For this review, use the dimensioned drawing (mm, ordinates from the lowest corner) and the shaded views. A direction names the side the tool comes from. Round coordinates to 2 decimals unless told otherwise and drop trailing zeros. Order: outer loops, then holes, each group sorted by start corner. A loop starts at its lowest first (then second) coordinate and runs counter-clockwise, first axis right, second up. Notation, with made-up numbers: M 12.25,83 L 70.25,83 A23 ccw 70.25,120 Z; hole C 1.25,-31 d7. An arc over 180 degrees is marked long. Use a Markdown table: item, result. Add a question column.
1. Consider section A-A on z = 4.15. State the section outline as (x, y) points (1 decimal), then the cut area to 3 significant figures.
2. Consider section B-B on z = 0.8. State the section outline as (x, y) points (1 decimal), then the cut area to 3 significant figures.
3. The part is to be moulded in two halves that separate along X. For the marked faces 3, 4 and 5, say which applies: +X half, -X half, draft (parallel to the pull), parting line (faces both ways), or undercut.
4. For the marked faces 1 and 2, list the 3-axis set-ups (+Z, -Z, +X, -X, +Y, -Y) from which the entire face can be reached by the end or side of a thin tool; tool diameter is ignored.
5. To check wall thickness, follow probe 1 along Y at (x, z) = (11, 4.3); probe 2 along Z at (x, y) = (9.75, 2) (1 decimal). State the ranges of each line that lie inside material, in increasing order.
6. Insertion check: P1, Ø1.5, axis at y = 5.5, z = 2.5, coming from the -X side; P2, Ø2, axis at x = 5.5, y = 11.5, coming from the +Z side. Each pin has a flat end and moves straight along its axis. Give the tip position at first contact, or say it passes through.
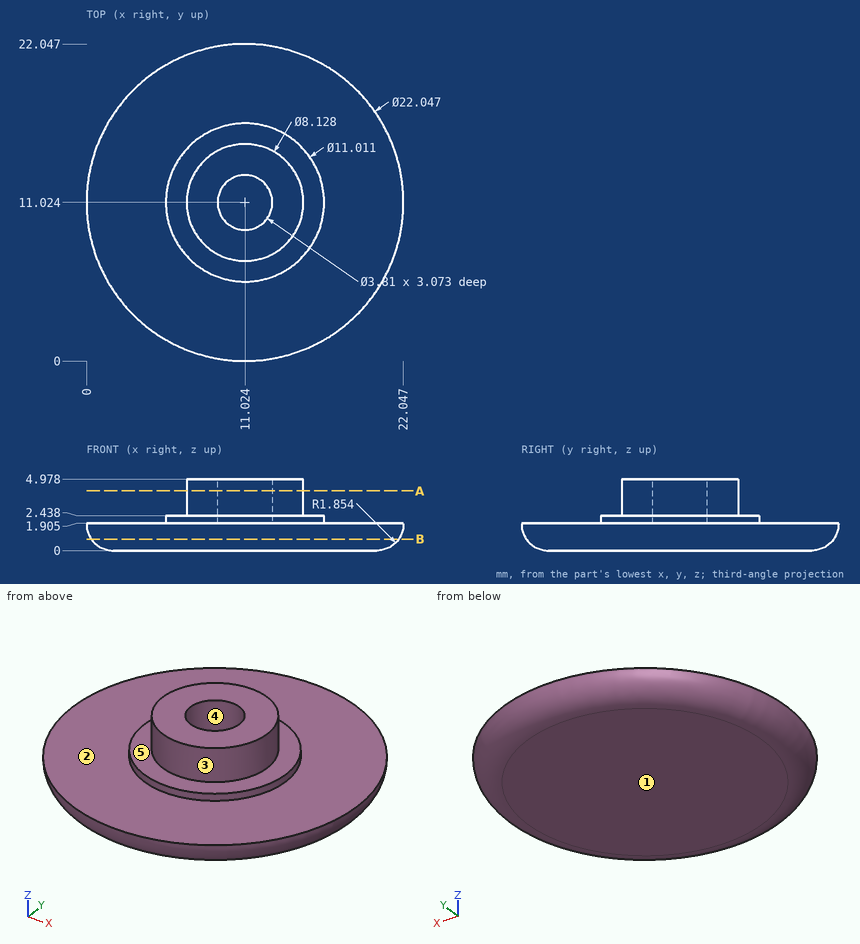
Answer block:
| question | item | result |
|---|---|---|
| 1 | outline | C 11,11 d8.1; hole C 11,11 d3.8 |
| 1 | area | 40.5 mm^2 |
| 2 | outline | C 11,11 d21.4 |
| 2 | area | 359 mm^2 |
| 3 | face 3 | parting line |
| 3 | face 4 | undercut |
| 3 | face 5 | draft |
| 4 | face 1 | -Z, +X, -X, +Y, -Y |
| 4 | face 2 | +Z |
| 5 | probe 1 | 6.96 to 9.12, 12.93 to 15.09 |
| 5 | probe 2 | 0 to 1.9 |
| 6 | P1 | x = 1.23 |
| 6 | P2 | z = 2.44 |
